The model under review builds one solid part; all positions refer to its coordinate system, in mm. Round coordinates to 2 decimals unless told otherwise and drop trailing zeros. Write each loop counter-clockwise with the first axis right and the second up, starting at its lowest first coordinate (ties: lowest second). Pieces come first, ordered by that corner, then holes. Notation, with made-up numbers: M -10.75,-24.75 L 10.25,-24.75 A21 cw 10.25,-18.75 Z; hole C -22,-10.75 d10. An arc over 180 degrees is marked long. One line per item, written item: value. Start each with the question number.
1) For P1, Ø1.5, axis at x = 35, z = -30.5, coming from the -Y side; P2, Ø0.9, axis at x = -47, y = 1, coming from the -Z side; P3, Ø2.5, axis at x = -47.5, z = -3.5, coming from the +Y side; P4, Ø1.5, axis at y = 2, z = -41, coming from the -X side, all flat-tipped, find the tip position at first contact; note any pin that passes through.
2) Take a section at C-C, the plane x = 30. Write out the cut boundary in (y, z).
3) Take a section at A-A, the plane x = 47.5. Write out the cut boundary in (y, z), and give its area (3 significant figures).
4) Take a section at B-B, the plane z = -3.5. Write out the cut boundary in (x, y).
5) Take a section at D-D, the plane z = -41.5. Write out the cut boundary in (x, y), and give its area (3 significant figures).
6) Wall thickness on probe 1 along X at (y, z) = (0.95, -3.5); probe 2 along X at (y, z) = (0.9, -41.5); probe 3 along X at (y, z) = (2.25, 5): over which ranges is each line inside the solid? List them lowest first.
from build123d import *

# Parameters (mm, degrees)
EXTRUDE_1_DEPTH     = 3
SKETCH_2_R          = 2.25
SKETCH_2_R_2        = 1.7
CUT_EXTRUDE_1_DEPTH = 3
FILLET_1_R          = 2


with BuildPart() as part:
    # 草图1 → 凸台-拉伸1 (new body)
    with BuildSketch(Plane(origin=(0, 0, 0), x_dir=(1, 0, 0), z_dir=(0, 1, 0))):
        Polygon((42.5, -31.5), (52.5, -31.5), (52.5, 31.5), (35, 31.5), (35, 46.5), (25, 46.5), (25, 31.5), (-25, 31.5), (-25, 46.5), (-35, 46.5), (-35, 31.5), (-52.5, 31.5), (-52.5, -31.5), (-42.5, -31.5), (-42.5, 21.5), (42.5, 21.5), align=None)
    extrude(amount=EXTRUDE_1_DEPTH)

    # 草图2 → 切除-拉伸1 (cut)
    with BuildSketch(Plane(origin=(0, 3, 0), x_dir=(1, 0, 0), z_dir=(0, 1, 0))):
        with Locations(Location((-47.5, -21.5, 0), (0, 0, 270))):
            Circle(SKETCH_2_R)
        with Locations(Location((-47.5, 3.5, 0), (0, 0, 270))):
            Circle(SKETCH_2_R)
        with Locations(Location((-30, 41.5, 0), (0, 0, 270))):
            Circle(SKETCH_2_R_2)
        with Locations(Location((47.5, -21.5, 0), (0, 0, 90))):
            Circle(SKETCH_2_R)
        with Locations(Location((47.5, 3.5, 0), (0, 0, 90))):
            Circle(SKETCH_2_R)
        with Locations(Location((30, 41.5, 0), (0, 0, 90))):
            Circle(SKETCH_2_R_2)
    extrude(amount=-CUT_EXTRUDE_1_DEPTH, mode=Mode.SUBTRACT)

    # 圆角1
    fillet_1_edges = [part.edges().sort_by_distance(p)[0] for p in [
        (52.5, 1.5, -31.5),
        (52.5, 1.5, 31.5),
        (42.5, 1.5, 31.5),
        (42.5, 1.5, -21.5),
        (-42.5, 1.5, -21.5),
        (-42.5, 1.5, 31.5),
        (-52.5, 1.5, 31.5),
        (-52.5, 1.5, -31.5),
        (-35, 1.5, -31.5),
        (-35, 1.5, -46.5),
        (-25, 1.5, -46.5),
        (-25, 1.5, -31.5),
        (25, 1.5, -31.5),
        (25, 1.5, -46.5),
        (35, 1.5, -46.5),
        (35, 1.5, -31.5),
    ]]
    fillet(fillet_1_edges, radius=FILLET_1_R)


solid = part.part
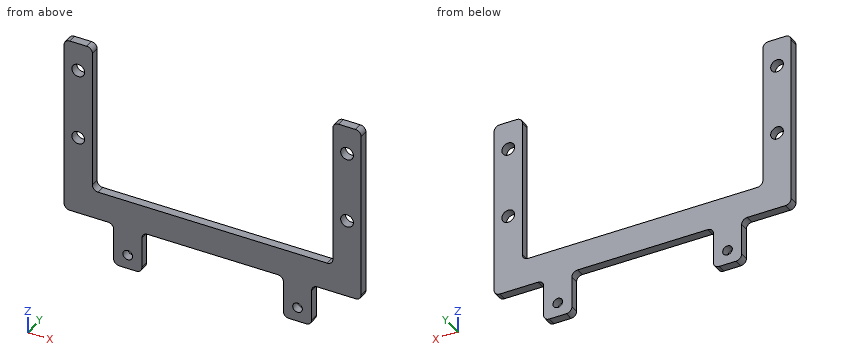
Checked values:
1. P1: stops at y = 0
1. P2: stops at z = -31.5
1. P3: passes through
1. P4: stops at x = -35
2. outline: M 0,-46.5 L 3,-46.5 L 3,-43.2 L 0,-43.2 Z; M 0,-39.8 L 3,-39.8 L 3,-21.5 L 0,-21.5 Z
3. outline: M 0,-31.5 L 3,-31.5 L 3,-5.75 L 0,-5.75 Z; M 0,-1.25 L 3,-1.25 L 3,19.25 L 0,19.25 Z; M 0,23.75 L 3,23.75 L 3,31.5 L 0,31.5 Z
3. area: 162 mm2
4. outline: M -52.5,0 L -49.75,0 L -49.75,3 L -52.5,3 Z; M -45.25,0 L -42.5,0 L -42.5,3 L -45.25,3 Z; M 42.5,0 L 45.25,0 L 45.25,3 L 42.5,3 Z; M 49.75,0 L 52.5,0 L 52.5,3 L 49.75,3 Z
5. outline: M -35,0 L -31.7,0 L -31.7,3 L -35,3 Z; M -28.3,0 L -25,0 L -25,3 L -28.3,3 Z; M 25,0 L 28.3,0 L 28.3,3 L 25,3 Z; M 31.7,0 L 35,0 L 35,3 L 31.7,3 Z
5. area: 39.6 mm2
6. probe 1: x = -52.5 to -49.75, -45.25 to -42.5, 42.5 to 45.25, 49.75 to 52.5
6. probe 2: x = -35 to -31.7, -28.3 to -25, 25 to 28.3, 31.7 to 35
6. probe 3: x = -52.5 to -42.5, 42.5 to 52.5
